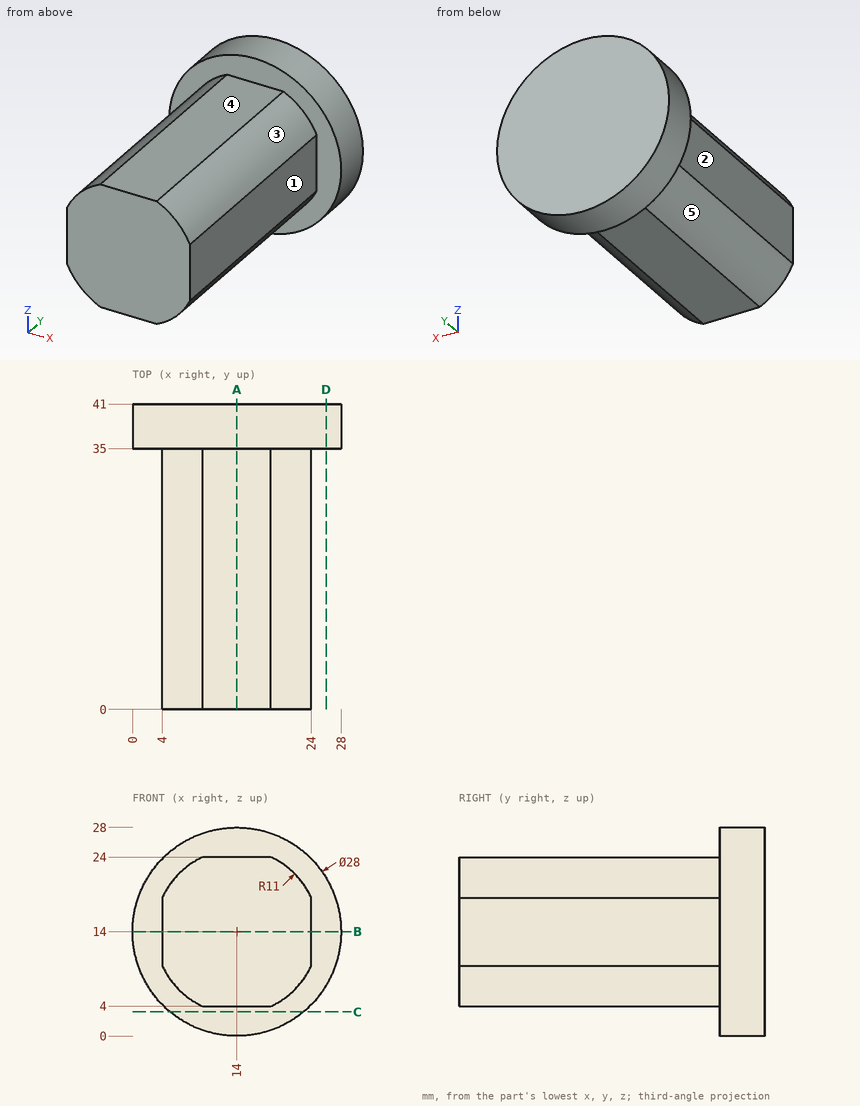
Answer from the drawing. Dimensions are ordinates in mm from the lowest x, y and z of the part. A direction names the side the tool comes from. Give positions to 0.01 mm unless a question says otherwise; leave off trailing zeros. Order: outer loops, then holes, each group sorted by start corner. A loop starts at its lowest first (then second) coordinate and runs counter-clockwise, first axis right, second up. Notation, with made-up numbers: (-35.5, 19) -> (13.5, 19) arc R25 cw to (13.5, 36) -> close; hole circle Ø5 at (47.5, 29). An arc over 180 degrees is marked (long way). Answer as a JSON object with one key per item and string values. Group by question number.
1. Section C-C on z = 3.25 is taken. Determine the outline of the cut face in (x, y), plus the area to 3 significant figures.
2. A tool of negligible diameter and unlimited length cuts with its end or side. For the marked faces 1, 2, 3, 4 and 5, from which of +Z, -Z, +X, -X, +Y, -Y can it reach the whole face along a straight path? Write none if from no direction.
3. Section D-D on x = 26 is taken. Determine the outline of the cut face in (y, z), plus the area to 3 significant figures.
4. Consider line 1 along Z through (x, y) = (11.5, 32); line 2 along Y through (x, z) = (1.5, 12). Determine where each line is inside the solid, lowest interval first. Write a range as [from, to].
5. Section A-A on x = 14 is taken. Determine the outline of the cut face in (y, z).
6. Section B-B on z = 14 is taken. Determine the outline of the cut face in (x, y), plus the area to 3 significant figures.
7. Flat-ended cylindrical pins translate along their axes: pin 1 Ø5 at (y, z) = (12, 3.5) entering from +X; pin 2 Ø10 at (x, y) = (12.5, 26) entering from +Z; pin 3 Ø1 at (x, y) = (9, 8) entering from -Z; pin 4 Ø3 at (x, z) = (15, 10.5) entering from -Y. Find the tip coordinate at first contact, or state that the pin passes through.
Result sheet:
{
 "1": {"outline": "(5.03, 35) -> (22.97, 35) -> (22.97, 41) -> (5.03, 41) -> close", "area": "108 mm^2"},
 "2": {"face 1": "+Z, -Z, +X, -Y", "face 2": "+Z, -Z, -X, -Y", "face 3": "+Z, +X, -Y", "face 4": "+Z, +X, -X, -Y", "face 5": "-Z, -X, -Y"},
 "3": {"outline": "(35, 6.79) -> (41, 6.79) -> (41, 21.21) -> (35, 21.21) -> close", "area": "86.5 mm^2"},
 "4": {"line 1": "z = [4, 24]", "line 2": "y = [35, 41]"},
 "5": {"outline": "(0, 4) -> (35, 4) -> (35, 0) -> (41, 0) -> (41, 28) -> (35, 28) -> (35, 24) -> (0, 24) -> close"},
 "6": {"outline": "(0, 35) -> (4, 35) -> (4, 0) -> (24, 0) -> (24, 35) -> (28, 35) -> (28, 41) -> (0, 41) -> close", "area": "868 mm^2"},
 "7": {"pin 1": "stops at x = 21.55", "pin 2": "stops at z = 24", "pin 3": "stops at z = 4", "pin 4": "stops at y = 0"}
}
